from build123d import *

# Parameters (mm, degrees)
IZIM2_W                     = 624.83438286
IZIM2_H                     = 493.118424104
Y_KSEKLIK_EKSTR_ZYON1_DEPTH = 500
IZIM4_R                     = 100
Y_KSEKLIK_EKSTR_ZYON2_DEPTH = 35
IZIM5_W                     = 975.967830922
IZIM5_H                     = 10.395315862
Y_KSEKLIK_EKSTR_ZYON3_DEPTH = 500
IZIM6_W                     = 317.202351564
IZIM6_H                     = 374.704466417
Y_KSEKLIK_EKSTR_ZYON4_DEPTH = 500
KES_EKSTR_ZYON1_DEPTH       = 500
KES_EKSTR_ZYON2_DEPTH       = 500
KES_EKSTR_ZYON3_DEPTH       = 500
IZIM11_R                    = 100
Y_KSEKLIK_EKSTR_ZYON5_DEPTH = 35
IZIM12_W                    = 466.303391348
IZIM12_H                    = 163.89871841
KES_EKSTR_ZYON4_DEPTH       = 35
IZIM17_W                    = 464.870730912
IZIM17_H                    = 199.827267797
KES_EKSTR_ZYON7_DEPTH       = 35
IZIM20_W                    = 465.660425645
IZIM20_H                    = 104.591429086
KES_EKSTR_ZYON8_DEPTH       = 35
IZIM21_W                    = 463.56331291
IZIM21_H                    = 33.15833205
KES_EKSTR_ZYON9_DEPTH       = 35
IZIM22_W                    = 465.770217683
IZIM22_H                    = 55.70279957
KES_EKSTR_ZYON10_DEPTH      = 35
IZIM23_W                    = 466.303391348
IZIM23_H                    = 30.655819637
KES_EKSTR_ZYON11_DEPTH      = 60
IZIM25_W                    = 26.274086754
IZIM25_H                    = 211.571078613
Y_KSEKLIK_EKSTR_ZYON6_DEPTH = 500
IZIM27_W                    = 465.215365456
IZIM27_H                    = 190.357875177
KES_EKSTR_ZYON12_DEPTH      = 60
IZIM28_R                    = 100
Y_KSEKLIK_EKSTR_ZYON7_DEPTH = 35


with BuildPart() as part:
    # Çizim2 → Yükseklik-Ekstrüzyon1 (new body)
    with BuildSketch(Plane(origin=(0, 0, 0), x_dir=(0, 0, -1), z_dir=(1, 0, 0))):
        with Locations((945.419542605, 684.894087956)):
            Rectangle(IZIM2_W, IZIM2_H)
    extrude(amount=-Y_KSEKLIK_EKSTR_ZYON1_DEPTH)

    # Çizim4 → Yükseklik-Ekstrüzyon2 (add)
    with BuildSketch(Plane(origin=(0, 0, 0), x_dir=(0, 0, -1), z_dir=(1, 0, 0))):
        with Locations((1137.354295612, 438.334875904)):
            Circle(IZIM4_R)
    extrude(amount=Y_KSEKLIK_EKSTR_ZYON2_DEPTH)

    # Çizim5 → Yükseklik-Ekstrüzyon3 (add)
    with BuildSketch(Plane(origin=(0, 0, 0), x_dir=(0, 0, -1), z_dir=(1, 0, 0))):
        with Locations((769.852818574, 433.137217973)):
            Rectangle(IZIM5_W, IZIM5_H)
    extrude(amount=-Y_KSEKLIK_EKSTR_ZYON3_DEPTH)

    # Çizim6 → Yükseklik-Ekstrüzyon4 (add)
    with BuildSketch(Plane(origin=(0, 0, 0), x_dir=(0, 0, -1), z_dir=(1, 0, 0))):
        with Locations((440.470078895, 615.291793251)):
            Rectangle(IZIM6_W, IZIM6_H)
    extrude(amount=-Y_KSEKLIK_EKSTR_ZYON4_DEPTH)

    # Çizim7 → Kes-Ekstrüzyon1 (cut)
    with BuildSketch(Plane(origin=(0, 0, 0), x_dir=(0, 0, -1), z_dir=(1, 0, 0))):
        Polygon((281.868903113, 802.644026459), (345.819234143, 802.644026459), (281.868903113, 615.29179325), align=None)
    extrude(amount=-KES_EKSTR_ZYON1_DEPTH, mode=Mode.SUBTRACT)

    # Çizim8 → Kes-Ekstrüzyon2 (cut)
    with BuildSketch(Plane(origin=(0, 0, 0), x_dir=(0, 0, -1), z_dir=(1, 0, 0))):
        Polygon((367.032437579, 781.430823023), (305.46881178, 612.286151281), (305.46881178, 499.123252309), (345.819234143, 499.123252309), (387.007160993, 612.286151281), (582.392266599, 612.286151281), (582.392266599, 781.430823023), align=None)
    extrude(amount=-KES_EKSTR_ZYON2_DEPTH, mode=Mode.SUBTRACT)

    # Çizim10 → Kes-Ekstrüzyon3 (cut)
    with BuildSketch(Plane(origin=(0, 0, 0), x_dir=(0, 0, -1), z_dir=(1, 0, 0))):
        Polygon((599.071254677, 438.334875904), (356.541223106, 438.334875904), (408.220364428, 591.072947846), (599.071254677, 591.072947846), align=None)
    extrude(amount=-KES_EKSTR_ZYON3_DEPTH, mode=Mode.SUBTRACT)

    # Çizim11 → Yükseklik-Ekstrüzyon5 (add)
    with BuildSketch(Plane(origin=(0, 0, 0), x_dir=(0, 0, -1), z_dir=(1, 0, 0))):
        with Locations((431.321316174, 427.939560042)):
            Circle(IZIM11_R)
    extrude(amount=Y_KSEKLIK_EKSTR_ZYON5_DEPTH)

    # Çizim12 → Kes-Ekstrüzyon4 (cut)
    with BuildSketch(Plane(origin=(0, -21.964844226, -64.349355999), x_dir=(1, 0, 0), z_dir=(0, 0.323037077, 0.94638631))):
        with Locations((-250, 772.34079435)):
            Rectangle(IZIM12_W, IZIM12_H)
    extrude(amount=-KES_EKSTR_ZYON4_DEPTH, mode=Mode.SUBTRACT)

    # Çizim17 → Kes-Ekstrüzyon7 (cut)
    with BuildSketch(Plane(origin=(0, 612.286151281, 0), x_dir=(1, 0, 0), z_dir=(0, 1, 0))):
        with Locations((-250, 482.478632701)):
            Rectangle(IZIM17_W, IZIM17_H)
    extrude(amount=-KES_EKSTR_ZYON7_DEPTH, mode=Mode.SUBTRACT)

    # Çizim20 → Kes-Ekstrüzyon8 (cut)
    with BuildSketch(Plane(origin=(0, -52.757830226, -144.950947246), x_dir=(1, 0, 0), z_dir=(0, 0.342020143, 0.939692621))):
        with Locations((-250.321482852, 639.324434245)):
            Rectangle(IZIM20_W, IZIM20_H)
    extrude(amount=-KES_EKSTR_ZYON8_DEPTH, mode=Mode.SUBTRACT)

    # Çizim21 → Kes-Ekstrüzyon9 (cut)
    with BuildSketch(Plane(origin=(0, -52.757830226, -144.950947246), x_dir=(1, 0, 0), z_dir=(0, 0.342020143, 0.939692621))):
        with Locations((-249.003107825, 691.169166414)):
            Rectangle(IZIM21_W, IZIM21_H)
    extrude(amount=-KES_EKSTR_ZYON9_DEPTH, mode=Mode.SUBTRACT)

    # Çizim22 → Kes-Ekstrüzyon10 (cut)
    with BuildSketch(Plane(origin=(0, -63.217651249, -186.84022059), x_dir=(-1, 0, 0), z_dir=(0, -0.320502572, -0.947247645))):
        with Locations((250.835570057, 555.815526561)):
            Rectangle(IZIM22_W, IZIM22_H)
    extrude(amount=-KES_EKSTR_ZYON10_DEPTH, mode=Mode.SUBTRACT)

    # Çizim23 → Kes-Ekstrüzyon11 (cut)
    with BuildSketch(Plane(origin=(0, 499.123252309, 0), x_dir=(1, 0, 0), z_dir=(0, 1, 0))):
        with Locations((-250, 324.988840267)):
            Rectangle(IZIM23_W, IZIM23_H)
    extrude(amount=-KES_EKSTR_ZYON11_DEPTH, mode=Mode.SUBTRACT)

    # Çizim25 → Yükseklik-Ekstrüzyon6 (add)
    with BuildSketch(Plane(origin=(0, 0, 0), x_dir=(0, 0, -1), z_dir=(1, 0, 0))):
        with Locations((476.795697093, 696.858487153)):
            Rectangle(IZIM25_W, IZIM25_H)
    extrude(amount=-Y_KSEKLIK_EKSTR_ZYON6_DEPTH)

    # Çizim27 → Kes-Ekstrüzyon12 (cut)
    with BuildSketch(Plane.XY.offset(-463.658653716)):
        with Locations((-250.172317272, 686.251885435)):
            Rectangle(IZIM27_W, IZIM27_H)
    extrude(amount=-KES_EKSTR_ZYON12_DEPTH, mode=Mode.SUBTRACT)

    # Çizim28 → Yükseklik-Ekstrüzyon7 (add)
    with BuildSketch(Plane.ZY.offset(500)):
        with Locations((-431.321316174, 427.939560042)):
            Circle(IZIM28_R)
        with Locations((-1135.713642363, 438.334875904)):
            Circle(IZIM28_R)
    extrude(amount=Y_KSEKLIK_EKSTR_ZYON7_DEPTH)


solid = part.part
Source: CAD feature listing. Evaluate the final solid. Frame: model axes, mm. A direction names the side the tool comes from. Round coordinates to 2 decimals unless told otherwise and drop trailing zeros. Loops run counter-clockwise (first coordinate to the right, second up) from the corner with the lowest first, then second, coordinate; pieces in that order, holes last. Notation, with made-up numbers: M 5.25,52 L 23.25,52 A23 ccw 23.25,85 Z; hole C -19,66 d9. An arc over 180 degrees is marked long. Return JSON: item names as keys, results as strings. Group by question number.
1. Mould query, pull axis Y, two halves, no side actions, for faces 5 (the face through (17.255, 389.639, -523.696)), 6 (the face through (0, 602, -416)), 7 (the face through (-253.26, 782.25, -352.84)). Classes: released by +Y, released by -Y, zero draft, split by the parting line, or undercut.
2. Material intervals for line 1 along Y through (x, z) = (-16, -416); line 2 along Z through (x, y) = (-313, 482.5); line 3 along Z through (x, y) = (-218.5, 771.5), sorted ascending. Write a range as from..to.
3. Pin query (flat end, axial travel): pin 1 (20 mm diameter, centred on x = -135, z = -324.5, fed in from +Y); pin 2 (3 mm diameter, centred on y = 617.5, z = -808.5, fed in from -X); pin 3 (2 mm diameter, centred on x = -154, z = -835, fed in from -Y). Return the tip coordinate at first contact, or that it passes through.
4. Reachability of faces 1 (the face through (-482.435, 600, -423)), 2 (the face through (-483.152, 470, -321)), 3 (the face through (0, 390, -430)), 4 (the face through (-249, 591.073, -588)) from +Z, -Z, +X, -X, +Y, -Y: full face, straight path, thin tool, end or side. Return the list, or none.
5. Section query A-A on y = 394.5. Output: boundary loops of the cut face in (x, z), and give its area (3 significant figures).
6. Section query D-D on z = -983. Output: boundary loops of the cut face in (x, y), and give its area (3 significant figures).
7. Section query B-B on x = -178.5. Output: boundary loops of the cut face in (y, z), and give its area (3 significant figures).
Checks:
{
 "1": {"face 5": "split by the parting line", "face 6": "zero draft", "face 7": "undercut"},
 "2": {"line 1": "y = 427.94..438.33, 591.07..612.29, 781.43..802.64", "line 2": "z = -1257.84..-633, -309.66..-281.87", "line 3": "z = -1257.84..-633, -599.07..-582.39"},
 "3": {"pin 1": "stops at y = 439.12", "pin 2": "stops at x = -500", "pin 3": "stops at y = 427.94"},
 "4": {"face 1": "none", "face 2": "+Y", "face 3": "+Z, -Z, -Y", "face 4": "+X, -X"},
 "5": {"outline": "M -535,-1225.59 L -500,-1225.59 L -500,-1045.83 L -535,-1045.83 Z; M -535,-525.56 L -500,-525.56 L -500,-337.08 L -535,-337.08 Z; M 0,-1227.23 L 35,-1227.23 L 35,-1047.47 L 0,-1047.47 Z; M 0,-525.56 L 35,-525.56 L 35,-337.08 L 0,-337.08 Z", "area": "25,800 mm²"},
 "6": {"outline": "M -500,427.94 L 0,427.94 L 0,931.45 L -500,931.45 Z", "area": "252,000 mm²"},
 "7": {"outline": "M 427.94,-1257.84 L 931.45,-1257.84 L 931.45,-633 L 438.33,-633 L 438.33,-356.54 L 436.9,-356.05 L 442.22,-340.32 L 439.12,-340.32 L 439.12,-309.66 L 499.12,-309.66 L 499.12,-305.47 L 612.29,-305.47 L 623.8,-309.66 L 631.41,-287.37 L 615.29,-281.87 L 427.94,-281.87 Z; M 591.07,-599.07 L 802.64,-599.07 L 802.64,-345.82 L 786.52,-340.32 L 777.85,-365.73 L 781.43,-367.03 L 781.43,-582.39 L 591.07,-582.39 Z", "area": "332,000 mm²"}
}
